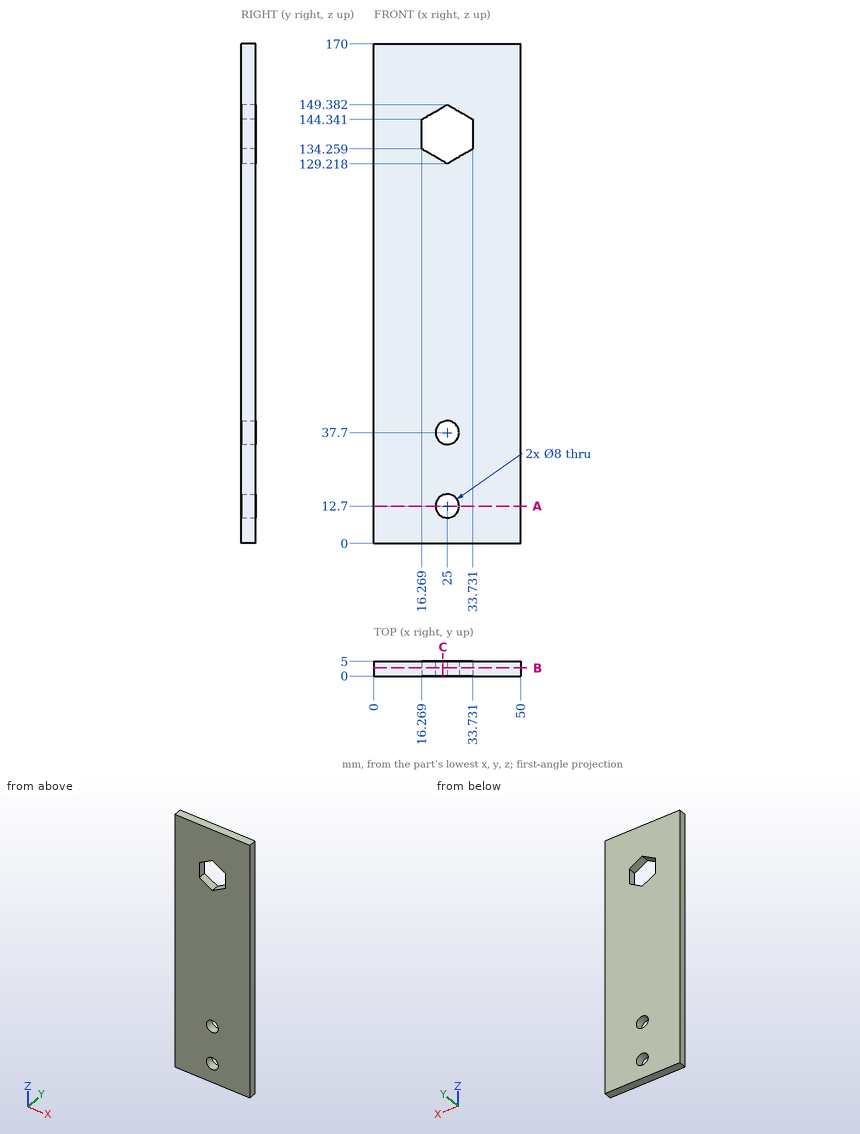
Here's the drawing with two shaded views (mm, measured from the low corner). I have some questions. Coordinates: 2 decimals unless noted, no trailing zeros. Write each loop counter-clockwise with the first axis right and the second up, starting at its lowest first coordinate (ties: lowest second). Pieces come first, ordered by that corner, then holes. Notation, with made-up numbers: M 67.25,34.25 L 94.25,34.25 A36 cw 94.25,73.25 Z; hole C 35,38 d2. An arc over 180 degrees is marked long. Answer as CSV lines item,"result". Start each with the question number.
1) I want a section at A-A, the plane z = 12.7. Please give me the cut outline in (x, y).
2) I want a section at B-B, the plane y = 2.8. Please give me the cut outline in (x, z).
3) I want a section at C-C, the plane x = 23.5. Please give me the cut outline in (y, z), and give its area (3 significant figures).
4) For P1, Ø12, axis at x = 14, z = 93.5, coming from the -Y side, with a flat end and sliding along its axis, tell me the tip position at first contact or that it passes through.
5) Please list where these lines run through material, in increasing order: line 1 (Z direction, x = 25, y = 3.65); line 2 (X direction, y = 1.8, z = 135); line 3 (Z direction, x = 26, y = 4.85) (1 decimal). Write a range as from..to.
Data:
1,outline,"M 0,0 L 21,0 L 21,5 L 0,5 Z; M 29,0 L 50,0 L 50,5 L 29,5 Z"
2,outline,"M 0,0 L 50,0 L 50,170 L 0,170 Z; hole M 16.27,134.26 L 25,129.22 L 33.73,134.26 L 33.73,144.34 L 25,149.38 L 16.27,144.34 Z; hole C 25,12.7 d8; hole C 25,37.7 d8"
3,outline,"M 0,0 L 5,0 L 5,8.99 L 0,8.99 Z; M 0,16.41 L 5,16.41 L 5,33.99 L 0,33.99 Z; M 0,41.41 L 5,41.41 L 5,130.08 L 0,130.08 Z; M 0,148.52 L 5,148.52 L 5,170 L 0,170 Z"
3,area,"684 mm^2"
4,P1,"stops at y = 0"
5,line 1,"z = 0..8.7, 16.7..33.7, 41.7..129.22, 149.38..170"
5,line 2,"x = 0..16.27, 33.73..50"
5,line 3,"z = 0..8.8, 16.6..33.8, 41.6..129.8, 148.8..170"
